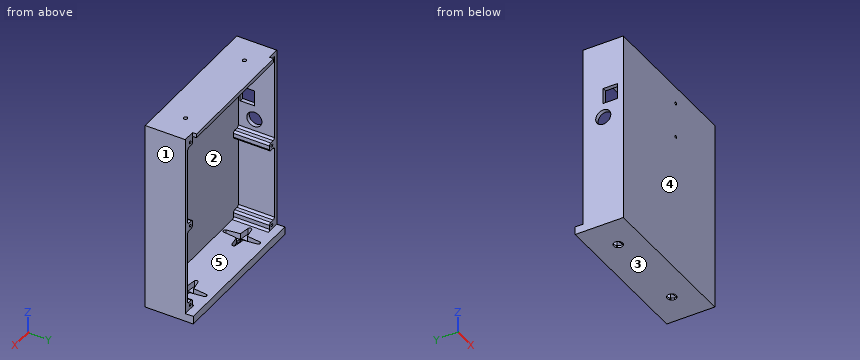
from build123d import *

# Parameters (mm, degrees)
SKETCH1_W                 = 120.65
SKETCH1_H                 = 152.4
BOSS_EXTRUDE1_DEPTH       = 3.175
SKETCH1_3_W               = 120.65
SKETCH1_3_H               = 152.4
SKETCH1_3_W_2             = 114.3
SKETCH1_3_H_2             = 142.875
BOSS_EXTRUDE2_DEPTH       = 38.1
SKETCH2_R                 = 1.5
CUT_EXTRUDE1_DEPTH        = 3.175
SKETCH3_R                 = 3.575
CUT_EXTRUDE8_DEPTH        = 4.7625
CUT_EXTRUDE9_DEPTH        = 163.546356849
CUT_EXTRUDE10_REACH       = 147.115
SKETCH4_R                 = 6
SKETCH4_W                 = 12.5
SKETCH4_H                 = 11.176
F_2_CLEARANCE_HOLE1_D     = 2.159
CUT_EXTRUDE11_DEPTH       = 3.175
SKETCH8_6_W               = 6.35
SKETCH8_6_H               = 142.875
CUT_EXTRUDE13_DEPTH       = 6.35
SKETCH9_W                 = 6.35
SKETCH9_H                 = 6.35
BOSS_EXTRUDE3_DEPTH       = 28.575
FILLET1_R                 = 1.5875
F_2_CLEARANCE_HOLE2_D     = 2.159
F_2_CLEARANCE_HOLE2_DEPTH = 12.7
F_2_CLEARANCE_HOLE2_TIP   = 0.648629038


with BuildPart() as part:
    # Sketch1 → Boss-Extrude1 (new body)
    with BuildSketch(Plane(origin=(0, 0, 0), x_dir=(1, 0, 0), z_dir=(0, 1, 0))):
        Rectangle(SKETCH1_W, SKETCH1_H)
    extrude(amount=BOSS_EXTRUDE1_DEPTH)

    # Sketch1<3> → Boss-Extrude2 (add)
    with BuildSketch(Plane(origin=(0, 0, 0), x_dir=(1, 0, 0), z_dir=(0, 1, 0))):
        Rectangle(SKETCH1_3_W, SKETCH1_3_H)
        with Locations((0, -1.5875)):
            Rectangle(SKETCH1_3_W_2, SKETCH1_3_H_2, mode=Mode.SUBTRACT)
    extrude(amount=BOSS_EXTRUDE2_DEPTH)

    # Sketch2 → Cut-Extrude1 (cut)
    with BuildSketch(Plane.XY.offset(76.2)):
        with Locations((38.825, 19.05)):
            Circle(SKETCH2_R)
    cut_extrude1 = extrude(amount=-CUT_EXTRUDE1_DEPTH, mode=Mode.SUBTRACT)

    # Sketch3 → Cut-Extrude8 (cut)
    with BuildSketch(Plane.XY.offset(-69.85)):
        with BuildLine():
            Line((33.833736344, 32.461656111), (32.677171347, 21.792446302))
            Line((32.677171347, 21.792446302), (24.788193615, 20.531189635))
            ThreePointArc((24.788193615, 20.531189635), (23.525, 19.05), (24.788193615, 17.568810365))
            Line((24.788193615, 17.568810365), (32.573739357, 16.324089971))
            Line((32.573739357, 16.324089971), (33.825, 5.8))
            ThreePointArc((33.825, 5.8), (35.325, 4.3), (36.825, 5.8))
            Line((36.825, 5.8), (38.076260643, 16.324089971))
            Line((38.076260643, 16.324089971), (45.861806385, 17.568810365))
            ThreePointArc((45.861806385, 17.568810365), (47.125, 19.05), (45.861806385, 20.531189635))
            Line((45.861806385, 20.531189635), (37.972828653, 21.792446302))
            Line((37.972828653, 21.792446302), (36.816263656, 32.461656111))
            ThreePointArc((36.816263656, 32.461656111), (35.325, 33.799999964), (33.833736344, 32.461656111))
        make_face()
        with Locations((35.325, 19.05)):
            Circle(SKETCH3_R, mode=Mode.SUBTRACT)
    cut_extrude8 = extrude(amount=-CUT_EXTRUDE8_DEPTH, mode=Mode.SUBTRACT)

    # Sketch3<8> → Cut-Extrude9 (cut, through all)
    with BuildSketch(Plane.XY.offset(-69.85)):
        with BuildLine():
            ThreePointArc((37.53121275, 16.23695), (37.852906743, 16.522093257), (38.13805, 16.84378725))
            ThreePointArc((38.13805, 16.84378725), (38.704147729, 17.882958602), (38.9, 19.05))
            ThreePointArc((38.9, 19.05), (38.671402302, 20.307861928), (38.014843843, 21.40485989))
            ThreePointArc((38.014843843, 21.40485989), (37.783724686, 21.645245252), (37.53121275, 21.86305))
            ThreePointArc((37.53121275, 21.86305), (35.325, 22.625), (33.11878725, 21.86305))
            ThreePointArc((33.11878725, 21.86305), (32.866275314, 21.645245252), (32.635156157, 21.40485989))
            ThreePointArc((32.635156157, 21.40485989), (31.751303585, 19.146534617), (32.51195, 16.84378725))
            ThreePointArc((32.51195, 16.84378725), (32.797093257, 16.522093257), (33.11878725, 16.23695))
            ThreePointArc((33.11878725, 16.23695), (35.325, 15.475), (37.53121275, 16.23695))
        make_face()
    cut_extrude9 = extrude(amount=-CUT_EXTRUDE9_DEPTH, mode=Mode.SUBTRACT)

    # Mirror1: Cut-Extrude1, Cut-Extrude8, Cut-Extrude9 across plane
    add(cut_extrude1.mirror(Plane(origin=(0, 0, 0), x_dir=(0, 0, 1), z_dir=(1, 0, 0))), mode=Mode.SUBTRACT)
    add(cut_extrude8.mirror(Plane(origin=(0, 0, 0), x_dir=(0, 0, 1), z_dir=(1, 0, 0))), mode=Mode.SUBTRACT)
    add(cut_extrude9.mirror(Plane(origin=(0, 0, 0), x_dir=(0, 0, 1), z_dir=(1, 0, 0))), mode=Mode.SUBTRACT)

    # Sketch4 → Cut-Extrude10 (cut, up to next)
    with BuildSketch(Plane(origin=(-57.15, 0, 0), x_dir=(0, 0, -1), z_dir=(1, 0, 0)), mode=Mode.PRIVATE) as cut_extrude10_sk1:
        with Locations((-14.095, 15.876)):
            Circle(SKETCH4_R)
    cut_extrude10_tool1 = extrude(cut_extrude10_sk1.sketch, amount=-CUT_EXTRUDE10_REACH, mode=Mode.PRIVATE) & part.part
    # Sketch4 → Cut-Extrude10 (cut, up to next)
    with BuildSketch(Plane(origin=(-57.15, 0, 0), x_dir=(0, 0, -1), z_dir=(1, 0, 0)), mode=Mode.PRIVATE) as cut_extrude10_sk2:
        with Locations((-31.775, 10.288)):
            Rectangle(SKETCH4_W, SKETCH4_H)
    cut_extrude10_tool2 = extrude(cut_extrude10_sk2.sketch, amount=-CUT_EXTRUDE10_REACH, mode=Mode.PRIVATE) & part.part
    add(cut_extrude10_tool1.solids().sort_by_distance((-57.15, 15.876, 14.095))[0], mode=Mode.SUBTRACT)
    add(cut_extrude10_tool2.solids().sort_by_distance((-57.15, 10.288, 31.775))[0], mode=Mode.SUBTRACT)

    # #2 Clearance Hole1 (through all)
    with Locations(Plane(origin=(8.85, 3.175, 62.6122), x_dir=(0, 0, 1), z_dir=(0, 1, 0))):
        with Locations((0, 0), (-28.0162, 0)):
            Hole(F_2_CLEARANCE_HOLE1_D / 2)

    # Sketch8 → Cut-Extrude11 (cut)
    with BuildSketch(Plane(origin=(0, 38.1, 0), x_dir=(1, 0, 0), z_dir=(0, 1, 0))):
        Polygon((-60.325, 69.85), (-60.325, -76.2), (60.325, -76.2), (60.325, 69.85), (57.15, 69.85), (57.15, -73.025), (-57.15, -73.025), (-57.15, 69.85), align=None)
    extrude(amount=-CUT_EXTRUDE11_DEPTH, mode=Mode.SUBTRACT)

    # Sketch8<6> → Cut-Extrude13 (cut)
    with BuildSketch(Plane(origin=(0, 38.1, 0), x_dir=(1, 0, 0), z_dir=(0, 1, 0))):
        Polygon((-60.325, 69.85), (-60.325, -76.2), (-50.8, -76.2), (-50.8, -73.025), (-57.15, -73.025), (-57.15, 69.85), align=None)
        with Locations((-53.975, -1.5875)):
            Rectangle(SKETCH8_6_W, SKETCH8_6_H)
        with Locations((53.975, -1.5875)):
            Rectangle(SKETCH8_6_W, SKETCH8_6_H)
        Polygon((50.8, -73.025), (50.8, -76.2), (60.325, -76.2), (60.325, 69.85), (57.15, 69.85), (57.15, -73.025), align=None)
    extrude(amount=-CUT_EXTRUDE13_DEPTH, mode=Mode.SUBTRACT)

    # Sketch9 → Boss-Extrude3 (add)
    with BuildSketch(Plane(origin=(0, 3.175, 0), x_dir=(1, 0, 0), z_dir=(0, 1, 0))):
        with Locations((-53.975, 0)):
            Rectangle(SKETCH9_W, SKETCH9_H)
        with Locations((53.975, 0)):
            Rectangle(SKETCH9_W, SKETCH9_H)
        with Locations((53.975, -69.85)):
            Rectangle(SKETCH9_W, SKETCH9_H)
        with Locations((-53.975, 66.675)):
            Rectangle(SKETCH9_W, SKETCH9_H)
        with Locations((53.975, 66.675)):
            Rectangle(SKETCH9_W, SKETCH9_H)
    extrude(amount=BOSS_EXTRUDE3_DEPTH)

    # Fillet1
    fillet1_edges = [part.edges().sort_by_distance(p)[0] for p in [
        (-57.15, 17.4625, -3.175),
        (-57.15, 17.4625, 3.175),
        (-50.8, 17.4625, 3.175),
        (-50.8, 17.4625, -3.175),
        (57.15, 17.4625, 3.175),
        (57.15, 17.4625, -3.175),
        (50.8, 17.4625, -3.175),
        (50.8, 17.4625, 3.175),
        (-57.15, 17.4625, -63.5),
        (-50.8, 17.4625, -63.5),
        (-50.8, 17.4625, -69.85),
        (57.15, 17.4625, 66.675),
        (50.8, 17.4625, 66.675),
        (50.8, 17.4625, 73.025),
        (57.15, 17.4625, -63.5),
        (50.8, 17.4625, -69.85),
        (50.8, 17.4625, -63.5),
    ]]
    fillet(fillet1_edges, radius=FILLET1_R)

    # #2 Clearance Hole2
    with Locations(Plane(origin=(0, 31.75, 0), x_dir=(1, 0, 0), z_dir=(0, 1, 0))):
        with Locations((53.975, 66.675), (53.975, -69.85), (53.975, 0), (-53.975, 0), (-53.975, 66.675)):
            Hole(F_2_CLEARANCE_HOLE2_D / 2, depth=F_2_CLEARANCE_HOLE2_DEPTH)
            with Locations((0, 0, -(F_2_CLEARANCE_HOLE2_DEPTH + F_2_CLEARANCE_HOLE2_TIP / 2))):  # 118° drill point
                Cone(0, F_2_CLEARANCE_HOLE2_D / 2, F_2_CLEARANCE_HOLE2_TIP, mode=Mode.SUBTRACT)


solid = part.part
Check sheet for the modelled part. Datum: model origin and axes. Units: mm. Face numbers are marked on the shaded views. A direction names the side the tool comes from. Round coordinates to 2 decimals unless told otherwise and drop trailing zeros. Order: outer loops, then holes, each group sorted by start corner. A loop starts at its lowest first (then second) coordinate and runs counter-clockwise, first axis right, second up.
(1) Cross-section at D-D, the plane y = 25. State how many separate pieces and enclosed holes the cut face has, and give its area (3 significant figures).
(2) Scan lines: probe 1 along X at (y, z) = (31.5, -37) (3 decimals); probe 2 along Z at (x, y) = (-19, 5) (3 decimals); probe 3 along X at (y, z) = (27, 69) (3 decimals). Record each from-to range of solid material in increasing order.
(3) Cross-section at B-B, the plane z = -16.5. Enter the section's corners in (x, y) (3 decimals).
(4) Go/stop test with flat-tipped pins: P1, Ø7, axis at y = 15.876, z = 14.095, coming from the -X side; P2, Ø12, axis at x = 8.5, z = -6, coming from the +Y side (3 decimals); P3, Ø2.5, axis at x = -59, z = 29, coming from the -Y side; P4, Ø2.5, axis at x = -59, z = 32, coming from the +Y side. Record where each tip stops, or that it passes through.
(5) Cross-section at A-A, the plane x = 20. Enter the section's corners in (y, z) (3 decimals), and give its area (3 significant figures).
(6) Cross-section at C-C, the plane z = 18.5. Enter the section's corners in (x, y) (3 decimals), and give its area (3 significant figures).
(7) Draft check along X on the marked faces 1, 2 and 3. Enter one of: pulls with the +X half, pulls with the -X half, needs draft (parallel to the pull), parting line crosses it, or undercut.
(8) Access from +Z, -Z, +X, -X, +Y, -Y to the whole of each face (thin tool, end or side, straight path). Record for the marked faces 4 and 5.
Check sheet entries:
1. separate pieces: 1
1. enclosed holes: 6
1. area: 2,200 mm2
2. probe 1: x = -60.325 to -57.15, 57.15 to 60.325
2. probe 2: z = -76.2 to -69.85, 73.025 to 76.2
2. probe 3: x = -60.325 to -57.15, 50.8 to 53.31, 54.64 to 60.325
3. outline: (-60.325, 0) - (60.325, 0) - (60.325, 31.75) - (57.15, 31.75) - (57.15, 3.175) - (-57.15, 3.175) - (-57.15, 31.75) - (-60.325, 31.75) - close
4. P1: stops at x = 57.15
4. P2: stops at y = 3.175
4. P3: stops at y = 0
4. P4: stops at y = 31.75
5. outline: (0, -76.2) - (38.1, -76.2) - (38.1, -69.85) - (3.175, -69.85) - (3.175, 73.025) - (34.925, 73.025) - (34.925, 76.2) - (0, 76.2) - close
5. area: 806 mm2
6. outline: (-60.325, 0) - (60.325, 0) - (60.325, 31.75) - (57.15, 31.75) - (57.15, 3.175) - (-57.15, 3.175) - (-57.15, 11.802) - (-60.325, 11.802) - close; (-60.325, 19.95) - (-57.15, 19.95) - (-57.15, 31.75) - (-60.325, 31.75) - close
6. area: 539 mm2
7. face 1: pulls with the +X half
7. face 2: undercut
7. face 3: needs draft
8. face 4: +Z, -Z, +X, -X, -Y
8. face 5: +Y
